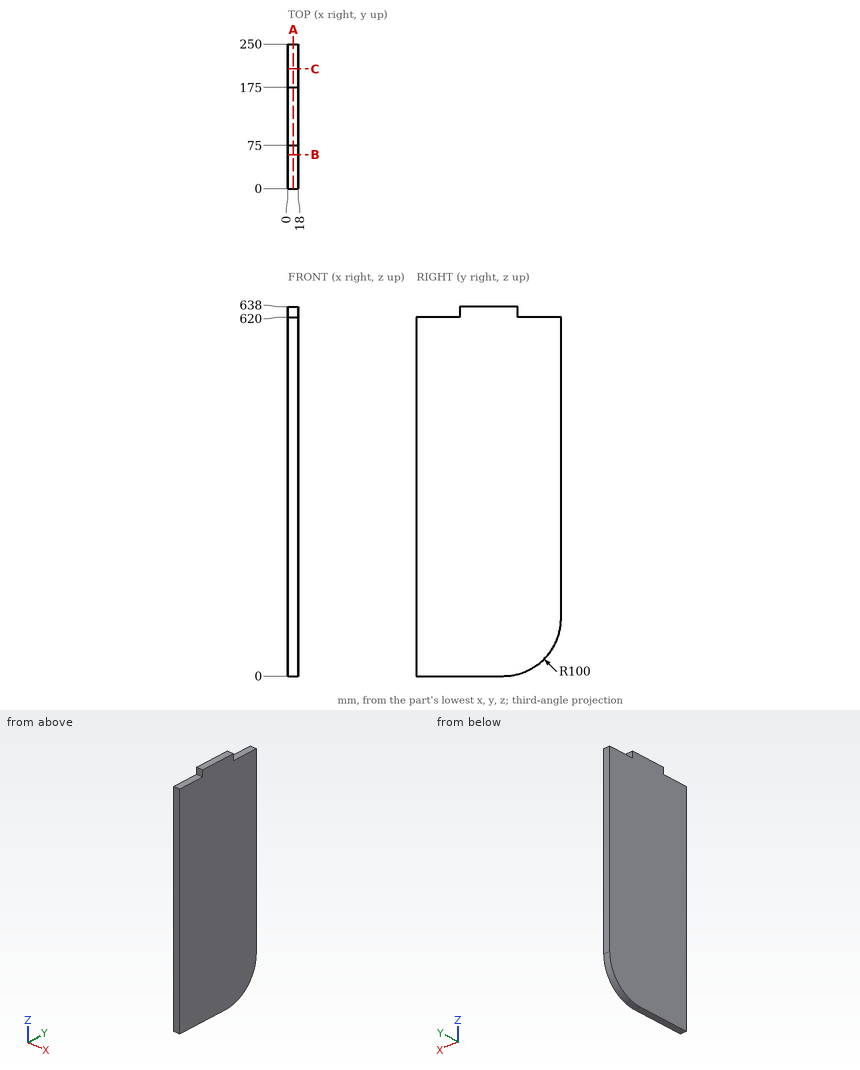
Here's the drawing with two shaded views (mm, measured from the low corner). I have some questions. Coordinates: 2 decimals unless noted, no trailing zeros. Write each loop counter-clockwise with the first axis right and the second up, starting at its lowest first coordinate (ties: lowest second). Pieces come first, ordered by that corner, then holes. Notation, with made-up numbers: (2, -10) -> (9, -10) arc R28 ccw to (9, 21) -> close; hole circle Ø4 at (44.5, 34). An arc over 180 degrees is marked (long way). Use a Markdown table: item, result. Add a question column.
(1) If we section it at A-A, the plane x = 9.25: Write out the boundary of the cut face in (y, z).
(2) If we section it at C-C, the plane y = 207: Write out the boundary of the cut face in (x, z), and give its area (3 significant figures).
(3) Please list where these lines run through material, in increasing order: line 1 (Z direction, x = 9.5, y = 44); line 2 (Z direction, x = 6.5, y = 207.5); line 3 (Y direction, x = 10.75, z = 78.5).
(4) I'm going to push flat-ended pins straight in: P1, Ø5, axis at x = 13, y = 31, coming from the +Z side; P2, Ø5.5, axis at x = 9.5, z = 631, coming from the -Y side. Where does each tip first touch, or does it pass through?
(5) If we section it at B-B, the plane y = 59: Write out the boundary of the cut face in (x, z).
Outcome:
| question | item | result |
|---|---|---|
| 1 | outline | (0, 0) -> (150, 0) arc R100 ccw to (250, 100) -> (250, 620) -> (175, 620) -> (175, 638) -> (75, 638) -> (75, 620) -> (0, 620) -> close |
| 2 | outline | (0, 17.84) -> (18, 17.84) -> (18, 620) -> (0, 620) -> close |
| 2 | area | 10,800 mm^2 |
| 3 | line 1 | z = 0 to 620 |
| 3 | line 2 | z = 18.18 to 620 |
| 3 | line 3 | y = 0 to 247.66 |
| 4 | P1 | stops at z = 620 |
| 4 | P2 | stops at y = 75 |
| 5 | outline | (0, 0) -> (18, 0) -> (18, 620) -> (0, 620) -> close |
